Could you check a few things on this model? Use its own coordinates, in mm. Face numbers are marked on the shaded views. Give positions to 0.01 mm unless a question says otherwise; leave off trailing zeros. Loops run counter-clockwise (first coordinate to the right, second up) from the corner with the lowest first, then second, coordinate; pieces in that order, holes last. Notation, with made-up numbers: (-0.75, 44) - (24.25, 44) arc R22 cw to (24.25, 80) - close; hole circle Ø3 at (50, 5.25). An arc over 180 degrees is marked (long way). Write each question's results on one line, items separated by ' | '. Start each with the question number.
(1) Suppose I cut it at A-A (y = 7.75). Please give me the cut outline in (x, z).
(2) Suppose I cut it at B-B (z = -8). Please give me the cut outline in (x, y).
(3) Suppose I cut it at C-C (x = -16). Please give me the cut outline in (y, z), and give its area (3 significant figures).
(4) I need wall thicknesses on line 1 (X direction, y = 12.5, z = 4.75); line 2 (Y direction, x = -53, z = 4.25); line 3 (X direction, y = 8.5, z = 6). Which ranges of each line are inside material? Lowest first, please.
(5) If we mould it in two halves opening along X, with no side actions, what happens to the marked faces 1 and 2? For each: released by +X, released by -X, zero draft, split by the parting line, or undercut.
(6) For pin 1 (2 mm diameter, centred on x = 48.25, y = 7.75, fed in from -Z); pin 2 (8 mm diameter, centred on y = 0.5, z = 3, fed in from -X); pin 3 (4 mm diameter, centred on x = 4, y = 0, fed in from -Z); pin 4 (4 mm diameter, centred on x = -48.5, z = -5.5, fed in from +Y), each with a flat end and sliding along its axis, tell me the tip position at first contact or that it passes through.
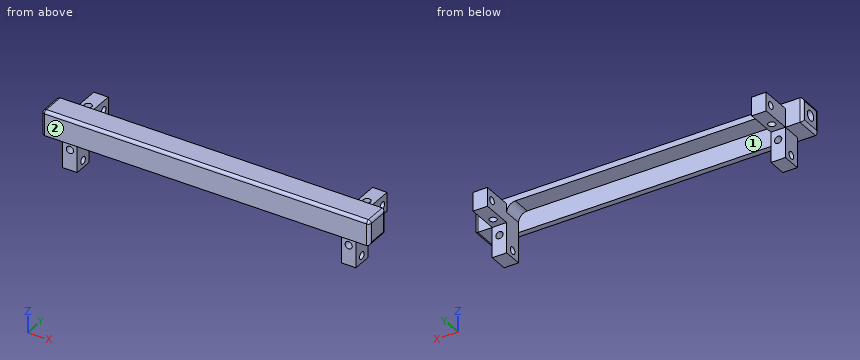
from build123d import *

# Parameters (mm, degrees)
SKETCH1_W                 = 113.5
SKETCH1_H                 = 8.5
BOSS_EXTRUDE1_DEPTH       = 8.5
BOSS_EXTRUDE2_DEPTH       = 5
BOSS_EXTRUDE3_DEPTH       = 5
SKETCH13_W                = 91.5
SKETCH13_H                = 6.5
CUT_EXTRUDE1_DEPTH        = 6.5
M3X0_5_TAPPED_HOLE1_D     = 2.5
M3X0_5_TAPPED_HOLE1_DEPTH = 7.5
M3X0_5_TAPPED_HOLE1_TIP   = 0.751075774
M3X0_5_TAPPED_HOLE2_D     = 2.5
M3X0_5_TAPPED_HOLE2_DEPTH = 5
M3X0_5_TAPPED_HOLE3_D     = 2.5
M3X0_5_TAPPED_HOLE3_DEPTH = 5
M3X0_5_TAPPED_HOLE4_D     = 2.5
M3X0_5_TAPPED_HOLE4_DEPTH = 7.5
M3X0_5_TAPPED_HOLE4_TIP   = 0.751075774
FILLET1_R                 = 1
FILLET2_R                 = 1
FILLET3_R                 = 1
FILLET4_R                 = 3
M3X0_5_TAPPED_HOLE5_D     = 2.5
M3X0_5_TAPPED_HOLE5_DEPTH = 7.5
M3X0_5_TAPPED_HOLE5_TIP   = 0.751075774
M3X0_5_TAPPED_HOLE6_D     = 2.5
M3X0_5_TAPPED_HOLE6_DEPTH = 7.5
M3X0_5_TAPPED_HOLE6_TIP   = 0.751075774
M3X0_5_TAPPED_HOLE7_D     = 2.5
M3X0_5_TAPPED_HOLE7_DEPTH = 7.5
M3X0_5_TAPPED_HOLE7_TIP   = 0.751075774
M3X0_5_TAPPED_HOLE9_D     = 2.5
M3X0_5_TAPPED_HOLE9_DEPTH = 7.5
M3X0_5_TAPPED_HOLE9_TIP   = 0.751075774
SKETCH43_W                = 10.5
SKETCH43_H                = 10.5
CUT_EXTRUDE3_DEPTH        = 110.01404726
F_8_36_TAPPED_HOLE1_D     = 3.4544
F_8_36_TAPPED_HOLE1_DEPTH = 12.1
F_8_36_TAPPED_HOLE1_TIP   = 1.037806461


with BuildPart() as part:
    # Sketch1 → Boss-Extrude1 (new body)
    with BuildSketch(Plane.XY):
        Rectangle(SKETCH1_W, SKETCH1_H)
    extrude(amount=BOSS_EXTRUDE1_DEPTH)

    # Sketch4 → Boss-Extrude2 (add)
    with BuildSketch(Plane(origin=(50.75, 0, 0), x_dir=(0, 0, -1), z_dir=(1, 0, 0))):
        Polygon((0, -2.25), (10.5, -2.25), (10.5, 14.75), (-6.5, 14.75), (-6.5, 4.25), (0, 4.25), align=None)
    extrude(amount=-BOSS_EXTRUDE2_DEPTH)

    # Sketch12 → Boss-Extrude3 (add)
    with BuildSketch(Plane.ZY.offset(50.75)):
        Polygon((6.5, 4.25), (6.5, 14.75), (-10.5, 14.75), (-10.5, -2.25), (0, -2.25), (0, 4.25), align=None)
    extrude(amount=-BOSS_EXTRUDE3_DEPTH)

    # Sketch13 → Cut-Extrude1 (cut)
    with BuildSketch(Plane(origin=(0, 4.25, 0), x_dir=(1, 0, 0), z_dir=(0, 1, 0))):
        with Locations((0, -3.25)):
            Rectangle(SKETCH13_W, SKETCH13_H)
    extrude(amount=-CUT_EXTRUDE1_DEPTH, mode=Mode.SUBTRACT)

    # M3x0.5 Tapped Hole1
    with Locations(Plane.XY.offset(6.5)):
        with Locations((-48.25, 7.75)):
            Hole(M3X0_5_TAPPED_HOLE1_D / 2, depth=M3X0_5_TAPPED_HOLE1_DEPTH)
            with Locations((0, 0, -(M3X0_5_TAPPED_HOLE1_DEPTH + M3X0_5_TAPPED_HOLE1_TIP / 2))):  # 118° drill point
                Cone(0, M3X0_5_TAPPED_HOLE1_D / 2, M3X0_5_TAPPED_HOLE1_TIP, mode=Mode.SUBTRACT)

    # M3x0.5 Tapped Hole2
    with Locations(Plane.ZY.offset(50.75)):
        with Locations((3.25, 12.25)):
            Hole(M3X0_5_TAPPED_HOLE2_D / 2, depth=M3X0_5_TAPPED_HOLE2_DEPTH)

    # M3x0.5 Tapped Hole3
    with Locations(Plane.ZY.offset(50.75)):
        with Locations((-8, 1)):
            Hole(M3X0_5_TAPPED_HOLE3_D / 2, depth=M3X0_5_TAPPED_HOLE3_DEPTH)

    # M3x0.5 Tapped Hole4
    with Locations(Plane.XZ.offset(2.25)):
        with Locations((-48.25, -3.5)):
            Hole(M3X0_5_TAPPED_HOLE4_D / 2, depth=M3X0_5_TAPPED_HOLE4_DEPTH)
            with Locations((0, 0, -(M3X0_5_TAPPED_HOLE4_DEPTH + M3X0_5_TAPPED_HOLE4_TIP / 2))):  # 118° drill point
                Cone(0, M3X0_5_TAPPED_HOLE4_D / 2, M3X0_5_TAPPED_HOLE4_TIP, mode=Mode.SUBTRACT)

    # Fillet1
    fillet1_edges = [part.edges().sort_by_distance(p)[0] for p in [
        (0, -4.25, 8.5),
    ]]
    fillet(fillet1_edges, radius=FILLET1_R)

    # Fillet2
    fillet2_edges = [part.edges().sort_by_distance(p)[0] for p in [
        (-56.75, 0.5, 8.5),
        (-56.75, 0, 0),
        (-56.75, 4.25, 4.25),
        (-56.75, -4.25, 3.75),
        (-56.75, -3.957106781, 8.207106781),
    ]]
    fillet(fillet2_edges, radius=FILLET2_R)

    # Fillet3
    fillet3_edges = [part.edges().sort_by_distance(p)[0] for p in [
        (56.75, 0, 0),
        (56.75, 4.25, 4.25),
        (56.75, 0.5, 8.5),
        (56.75, -4.25, 3.75),
        (56.75, -3.957106781, 8.207106781),
    ]]
    fillet(fillet3_edges, radius=FILLET3_R)

    # Fillet4
    fillet4_edges = [part.edges().sort_by_distance(p)[0] for p in [
        (-45.75, 1, 6.5),
        (45.75, 1, 6.5),
    ]]
    fillet(fillet4_edges, radius=FILLET4_R)

    # M3x0.5 Tapped Hole5
    with Locations(Plane.XY.offset(6.5)):
        with Locations((48.25, 7.75)):
            Hole(M3X0_5_TAPPED_HOLE5_D / 2, depth=M3X0_5_TAPPED_HOLE5_DEPTH)
            with Locations((0, 0, -(M3X0_5_TAPPED_HOLE5_DEPTH + M3X0_5_TAPPED_HOLE5_TIP / 2))):  # 118° drill point
                Cone(0, M3X0_5_TAPPED_HOLE5_D / 2, M3X0_5_TAPPED_HOLE5_TIP, mode=Mode.SUBTRACT)

    # M3x0.5 Tapped Hole6
    with Locations(Plane.XZ.offset(2.25)):
        with Locations((48.25, -3.5)):
            Hole(M3X0_5_TAPPED_HOLE6_D / 2, depth=M3X0_5_TAPPED_HOLE6_DEPTH)
            with Locations((0, 0, -(M3X0_5_TAPPED_HOLE6_DEPTH + M3X0_5_TAPPED_HOLE6_TIP / 2))):  # 118° drill point
                Cone(0, M3X0_5_TAPPED_HOLE6_D / 2, M3X0_5_TAPPED_HOLE6_TIP, mode=Mode.SUBTRACT)

    # M3x0.5 Tapped Hole7
    with Locations(Plane(origin=(50.75, 0, 0), x_dir=(0, 0, -1), z_dir=(1, 0, 0))):
        with Locations((8, 1)):
            Hole(M3X0_5_TAPPED_HOLE7_D / 2, depth=M3X0_5_TAPPED_HOLE7_DEPTH)
            with Locations((0, 0, -(M3X0_5_TAPPED_HOLE7_DEPTH + M3X0_5_TAPPED_HOLE7_TIP / 2))):  # 118° drill point
                Cone(0, M3X0_5_TAPPED_HOLE7_D / 2, M3X0_5_TAPPED_HOLE7_TIP, mode=Mode.SUBTRACT)

    # M3x0.5 Tapped Hole9
    with Locations(Plane(origin=(50.75, 0, 0), x_dir=(0, 0, -1), z_dir=(1, 0, 0))):
        with Locations((-3.25, 12.25)):
            Hole(M3X0_5_TAPPED_HOLE9_D / 2, depth=M3X0_5_TAPPED_HOLE9_DEPTH)
            with Locations((0, 0, -(M3X0_5_TAPPED_HOLE9_DEPTH + M3X0_5_TAPPED_HOLE9_TIP / 2))):  # 118° drill point
                Cone(0, M3X0_5_TAPPED_HOLE9_D / 2, M3X0_5_TAPPED_HOLE9_TIP, mode=Mode.SUBTRACT)

    # Sketch43 → Cut-Extrude3 (cut, through all)
    with BuildSketch(Plane.ZY.offset(50.75)):
        with Locations((-5.25, 9.5)):
            Rectangle(SKETCH43_W, SKETCH43_H)
    extrude(amount=-CUT_EXTRUDE3_DEPTH, mode=Mode.SUBTRACT)

    # #8-36 Tapped Hole1
    with Locations(Plane.ZY.offset(56.75)):
        with Locations((4.25, 0)):
            Hole(F_8_36_TAPPED_HOLE1_D / 2, depth=F_8_36_TAPPED_HOLE1_DEPTH)
            with Locations((0, 0, -(F_8_36_TAPPED_HOLE1_DEPTH + F_8_36_TAPPED_HOLE1_TIP / 2))):  # 118° drill point
                Cone(0, F_8_36_TAPPED_HOLE1_D / 2, F_8_36_TAPPED_HOLE1_TIP, mode=Mode.SUBTRACT)


solid = part.part
Output values:
1) outline: (-50.75, 0) - (-49.5, 0) - (-49.5, 6.5) - (-50.75, 6.5) - close; (-47, 0) - (-45.75, 0) - (-45.75, 6.5) - (-47, 6.5) - close; (45.75, 0) - (47, 0) - (47, 6.5) - (45.75, 6.5) - close; (49.5, 0) - (50.75, 0) - (50.75, 6.5) - (49.5, 6.5) - close
2) outline: (-50.75, -2.25) - (-45.75, -2.25) - (-45.75, -0.25) - (-50.75, -0.25) - close; (-50.75, 2.25) - (-45.75, 2.25) - (-45.75, 4.25) - (-50.75, 4.25) - close; (45.75, -2.25) - (50.75, -2.25) - (50.75, -0.25) - (45.75, -0.25) - close; (45.75, 2.25) - (50.75, 2.25) - (50.75, 4.25) - (45.75, 4.25) - close
3) outline: (-4.25, 0) - (-2.25, 0) - (-2.25, 6.5) - (4.25, 6.5) - (4.25, 8.5) - (-3.25, 8.5) arc R1 ccw to (-4.25, 7.5) - close | area: 29.8 mm2
4) line 1: -50.75 to -45.75, 45.75 to 50.75 | line 2: -4.25 to -1.73, 1.73 to 4.25 | line 3: -50.75 to -49.25, -47.25 to -45.75, 45.75 to 47.25, 49.25 to 50.75
5) face 1: undercut | face 2: zero draft
6) pin 1: through | pin 2: x = -56.75 | pin 3: z = 6.5 | pin 4: y = 4.25
